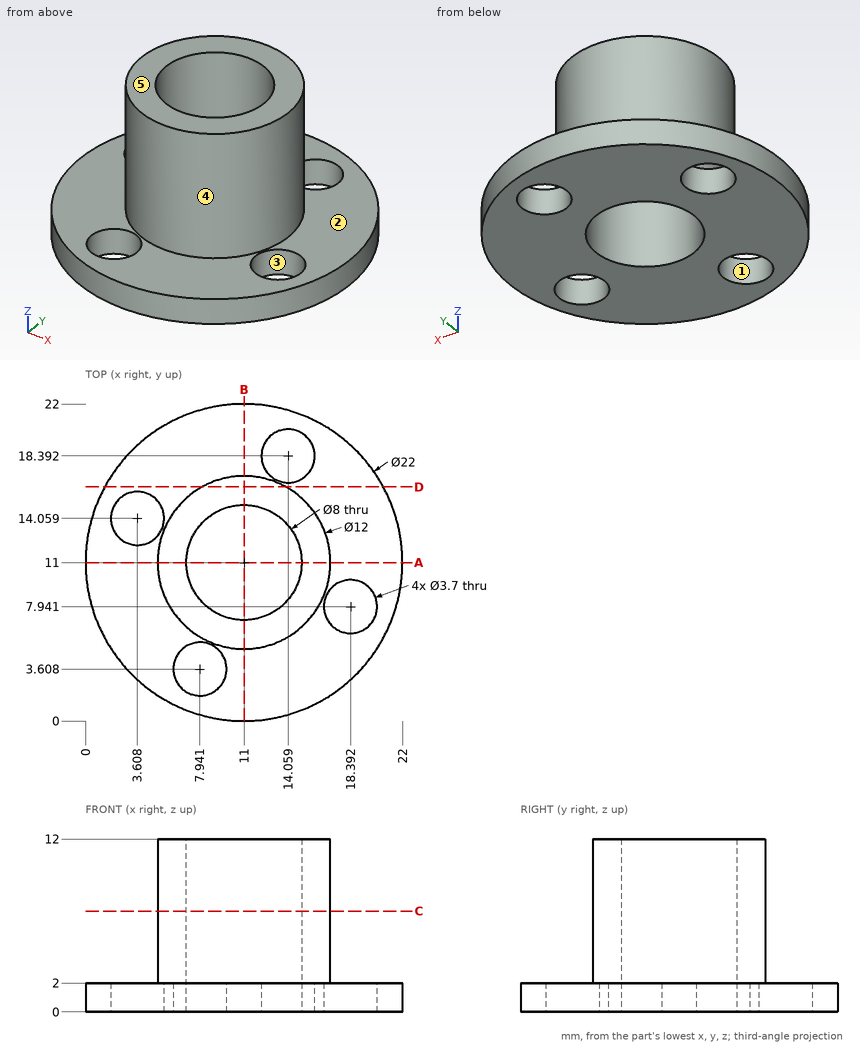
The drawing under review shows one solid part. Ordinate dimensions are in mm from its lowest x, y, z. A direction names the side the tool comes from. Give positions to 0.01 mm unless a question says otherwise; leave off trailing zeros. Write each loop counter-clockwise with the first axis right and the second up, starting at its lowest first coordinate (ties: lowest second). Pieces come first, ordered by that corner, then holes. Notation, with made-up numbers: (11, 15) -> (38, 15) arc R21 ccw to (38, 28) -> close; hole circle Ø11 at (3, 57). An arc over 180 degrees is marked (long way). Put each result on its own line as item: value.
(1) Tool access review of the marked faces 1 and 2: name each direction out of +Z, -Z, +X, -X, +Y, -Y from which nothing blocks a thin tool from reaching the whole face with its end or side.
Results are:
face 1: +Z, -Z
face 2: +Z
(2) We need section C-C, the plane z = 7. Give the boundary of the cut face in (x, y).
Results are:
outline: circle Ø12 at (11, 11); hole circle Ø8 at (11, 11)
(3) To check wall thickness, follow probe 1 along X at (y, z) = (12, 10.5) (1 decimal); probe 2 along X at (y, z) = (14.25, 7.5) (1 decimal); probe 3 along Y at (x, z) = (9, 5.75) (1 decimal). State the ranges of each line that lie inside material, in increasing order. Write a range as from..to.
Results are:
probe 1: 5.1..7.1, 14.9..16.9
probe 2: 6..8.7, 13.3..16
probe 3: 5.3..7.5, 14.5..16.7
(4) We need section A-A, the plane y = 11. Give the boundary of the cut face in (x, z).
Results are:
outline: (0, 0) -> (7, 0) -> (7, 12) -> (5, 12) -> (5, 2) -> (0, 2) -> close; (15, 0) -> (22, 0) -> (22, 2) -> (17, 2) -> (17, 12) -> (15, 12) -> close
(5) We need section D-D, the plane y = 16.25. Give the boundary of the cut face in (x, z) (1 decimal).
Results are:
outline: (1.3, 0) -> (20.7, 0) -> (20.7, 2) -> (13.9, 2) -> (13.9, 12) -> (8.1, 12) -> (8.1, 2) -> (1.3, 2) -> close
(6) The part is to be moulded in two halves that separate along Y. For the marked faces 3, 4 and 5, say which applies: pulls with the +Y half, pulls with the -Y half, needs draft (parallel to the pull), parting line crosses it, or undercut.
Results are:
face 3: undercut
face 4: parting line crosses it
face 5: needs draft
(7) For pin 1 Ø2 at (y, z) = (6.5, 9.5) entering from -X; pin 2 Ø5 at (y, z) = (18.5, 9.5) entering from -X (1 decimal); pin 3 Ø6 at (x, z) = (8, 7) entering from +Y, all flat-tipped, find the tip position at first contact; note any pin that passes through.
Results are:
pin 1: x = 6.13
pin 2: x = 7.7
pin 3: y = 17
